```python
from build123d import *

# Parameters (mm, degrees)
F_1_4_0_25_DIAMETER_HOLE1_D = 6.35
CIRPATTERN1_COUNT           = 8


with BuildPart() as part:
    # Sketch1 → Revolve1 (revolve)
    with BuildSketch(Plane.XY):
        Polygon((-12.7, 0), (-28.575, 0), (-50.8, -12.7), (-76.2, -12.7), (-76.2, -38.1), (-58.3057, -38.1), (-58.3057, -36.068), (-55.5625, -36.068), (-55.5625, -38.1), (-53.975, -38.1), (-53.975, -25.4), (-39.2557, -25.4), (-39.2557, -23.368), (-36.5125, -23.368), (-36.5125, -25.4), (-34.925, -25.4), (-34.925, -19.05), (-12.7, -6.35), align=None)
    revolve(axis=Axis((0, 0, 0), (0, 1, 0)))

    # 1_4 _0.25_ Diameter Hole1 (through all)
    with Locations(Plane(origin=(-66.675, 0, 0), x_dir=(0, 0, 1), z_dir=(0, 1, 0))):
        with Locations((0, 0)):
            f_1_4_0_25_diameter_hole1 = Hole(F_1_4_0_25_DIAMETER_HOLE1_D / 2)

    # CirPattern1: 1_4 _0.25_ Diameter Hole1 ×8 about axis
    cirpattern1_axis = Axis((0, 0, 0), (0, 1, 0))
    for i in range(1, CIRPATTERN1_COUNT):
        add(f_1_4_0_25_diameter_hole1.rotate(cirpattern1_axis, i * 360 / CIRPATTERN1_COUNT), mode=Mode.SUBTRACT)


solid = part.part
```
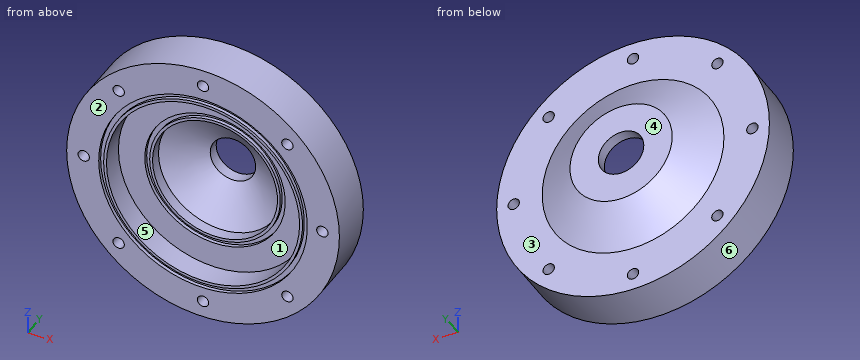
Check sheet for the modelled part. Datum: model origin and axes. Units: mm. Face numbers are marked on the shaded views. A direction names the side the tool comes from. Give positions to 0.01 mm unless a question says otherwise; leave off trailing zeros. One line per question, with ' | ' between items. Start each with the question number.
1. Gauge pin test, flat ends, axial feed: pin 1 Ø8.5 at (x, z) = (0, -66.675) entering from +Y; pin 2 Ø2 at (x, y) = (23, -24.5) entering from +Z; pin 3 Ø1.5 at (x, y) = (-51.5, -29.5) entering from -Z; pin 4 Ø4 at (x, z) = (-66.675, 0) entering from -Y. Record the tip position at first contact, or that the pin passes through.
2. Draft check along X on the marked faces 4, 5 and 6. Enter one of: released by +X, released by -X, zero draft, split by the parting line, or undercut.
3. Set-up check for the marked faces 1, 2 and 3: record each of +Z, -Z, +X, -X, +Y, -Y from which the full face is reachable in a straight line by a thin tool's end or side.
4. Cross-section at A-A, the plane y = -30. Give the number of separate pieces and of enclosed holes in the cut face, plus the area to 3 significant figures.
5. Material ranges on line 1 along Z through (x, y) = (0, -30.75) (3 decimals); line 2 along Z through (x, y) = (0, -23) (3 decimals); line 3 along X through (y, z) = (-17, 2), recorded low to high. Write a range as [from, to].
Check result:
1) pin 1: stops at y = -12.7 | pin 2: stops at z = 72.96 | pin 3: stops at z = -56.84 | pin 4: passes through
2) face 4: zero draft | face 5: undercut | face 6: split by the parting line
3) face 1: -Y | face 2: +Z, -Z, +X, -X, -Y | face 3: +Y
4) separate pieces: 1 | enclosed holes: 9 | area: 8,840 mm2
5) line 1: z = [-76.2, -69.85], [-63.5, -53.975], [53.975, 63.5], [69.85, 76.2] | line 2: z = [-76.2, -69.85], [-63.5, -34.925], [34.925, 63.5], [69.85, 76.2] | line 3: x = [-76.17, -69.14], [-64.21, -31.27], [31.27, 64.21], [69.14, 76.17]
